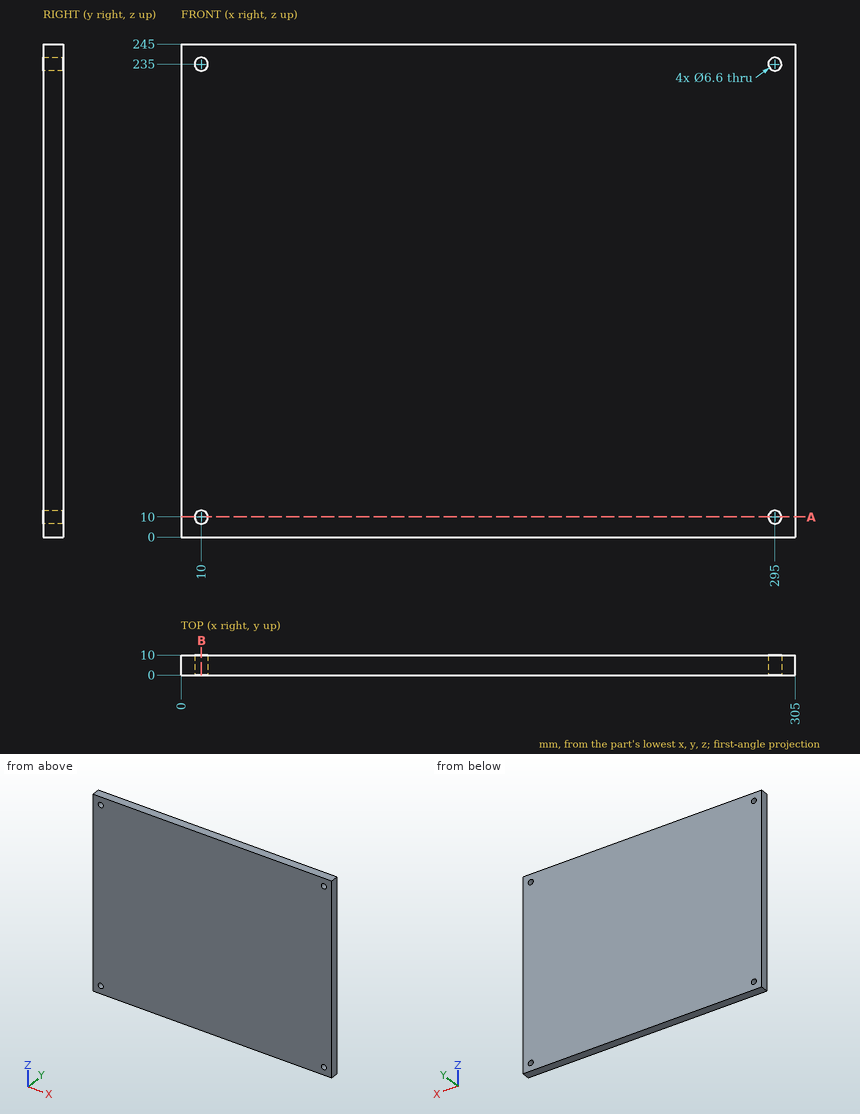
Could you check a few things on this drawing? It's one solid part, dimensions in mm from its lowest x, y, z. Coordinates: 2 decimals unless noted, no trailing zeros. Write each loop counter-clockwise with the first axis right and the second up, starting at its lowest first coordinate (ties: lowest second). Pieces come first, ordered by that corner, then holes. Notation, with made-up numbers: (10, -36) - (68, -36) arc R9 ccw to (68, -21) - close; hole circle Ø5 at (2.5, 36). An arc over 180 degrees is marked (long way). Put each result on its own line as item: value. Start each with the question number.
Q1. I want a section at B-B on x = 10. Write out the boundary of the cut face in (y, z), plus the area to 3 significant figures.
Q2. I'm going to push a flat-ended pin straight in: P1, Ø5.5, axis at x = 295, z = 10, coming from the +Y side. Where does the tip first touch, or does it pass through?
Q3. Please list where these lines run through material, in increasing order: L1, parallel to X at y = 7.75, z = 235; L2, parallel to Z at x = 10, y = 2; L3, parallel to X at y = 5.25, z = 232.5.
Q4. I want a section at A-A on z = 10. Write out the boundary of the cut face in (x, y).
Checks:
1. outline: (0, 0) - (10, 0) - (10, 6.7) - (0, 6.7) - close; (0, 13.3) - (10, 13.3) - (10, 231.7) - (0, 231.7) - close; (0, 238.3) - (10, 238.3) - (10, 245) - (0, 245) - close
1. area: 2,320 mm²
2. P1: through
3. L1: 0 to 6.7, 13.3 to 291.7, 298.3 to 305
3. L2: 0 to 6.7, 13.3 to 231.7, 238.3 to 245
3. L3: 0 to 7.85, 12.15 to 292.85, 297.15 to 305
4. outline: (0, 0) - (6.7, 0) - (6.7, 10) - (0, 10) - close; (13.3, 0) - (291.7, 0) - (291.7, 10) - (13.3, 10) - close; (298.3, 0) - (305, 0) - (305, 10) - (298.3, 10) - close
